Verification items for the finished model (mm, model axes). Give positions to 0.01 mm unless a question says otherwise; leave off trailing zeros. Order: outer loops, then holes, each group sorted by start corner. A loop starts at its lowest first (then second) coordinate and runs counter-clockwise, first axis right, second up. Notation, with made-up numbers: (55, -39) -> (73, -39) arc R18 cw to (73, -12) -> close; hole circle Ø9 at (-3, 67.25). An arc over 180 degrees is marked (long way). Return JSON: item names as keys, results as strings. Group by question number.
(1) Cross-section at B-B on y = 7.5. Enter the section's corners in (x, z) (1 decimal).
(2) Cross-section at A-A on z = 0. Enter the section's corners in (x, y), then the cut area to 3 significant figures.
(3) Thickness scan on line 1 along X through (y, z) = (8.5, -1); line 2 along Z through (x, y) = (-0.25, 5.75); line 3 along X through (y, z) = (9.75, -0.25). Record the ranges inside material, lowest first.
(4) Cross-section at D-D on x = -1.75. Enter the section's corners in (y, z).
(5) Release check for a two-part mould opening along Z. For faces 1 (the face through (1.578, 5.896, -2.784)), 2 (the face through (3.2, 6, 0)), 3 (the face through (-0.31, 5.9, -1.39)) record: pulls with the +Z half, pulls with the -Z half, needs draft (parallel to the pull), parting line crosses it, or undercut.
(6) Depth check by flat-ended pin: pin 1 Ø3 at (x, y) = (-2.5, 6.5) entering from -Z; pin 2 Ø2 at (y, z) = (1.5, -3) entering from +X; pin 3 Ø2 at (x, y) = (2.5, 6.5) entering from -Z. Enter the tip coordinate at first touch or a pass-through.
(7) Cross-section at C-C on x = 0.5. Enter the section's corners in (y, z), then the cut area to 3 significant figures.
Autodesk Inventor part; units mm, degrees
ref_plane "YZ Plane" through (0, 0, 0) normal (1, 0, 0) x (0, 1, 0)
ref_plane "XZ Plane" through (0, 0, 0) normal (0, 1, 0) x (-1, 0, 0)
ref_plane "XY Plane" through (0, 0, 0) normal (0, 0, 1) x (1, 0, 0)
sketch "Sketch1" plane through (0, 0, 0) normal (0, 1, 0) x (-1, 0, 0)
  line L0 (3.2, 1.8475) -> (3.2, -1.8475)
  line L1 (3.2, -1.8475) -> (0, -3.695)
  line L2 (0, -3.695) -> (-3.2, -1.8475)
  line L3 (-3.2, -1.8475) -> (-3.2, 1.8475)
  line L4 (-3.2, 1.8475) -> (0, 3.695)
  line L5 (0, 3.695) -> (3.2, 1.8475)
  point P0 (0, 0)
  point P1 (3.2, 0)
  point P2 (-3.2, 0)
  dimension "d0" = 6.4
  dimension "d1" = 120
  dimension "d2" = 6.4
extrude "Extrusion1" add sketch "Sketch1" along normal blind 11.96
sketch "Sketch3" plane through (0, 0, 0) normal (0, -1, 0) x (1, 0, 0)
  circle A0 centre (0, 0) radius 1.4224
  dimension "d8" = 2.8448
extrude "Extrusion3" cut sketch "Sketch3" against normal through all
properties part number "pc104standoffTEMP2" material "Stainless Steel"
Verdict:
{
 "1": {"outline": "(-3.2, -1.8) -> (0, -3.7) -> (3.2, -1.8) -> (3.2, 1.8) -> (0, 3.7) -> (-3.2, 1.8) -> close; hole circle Ø2.8 at (0, 0)"},
 "2": {"outline": "(-3.2, 0) -> (-1.42, 0) -> (-1.42, 11.96) -> (-3.2, 11.96) -> close; (1.42, 0) -> (3.2, 0) -> (3.2, 11.96) -> (1.42, 11.96) -> close", "area": "42.5 mm²"},
 "3": {"line 1": "-3.2 to -1.01, 1.01 to 3.2", "line 2": "-3.55 to -1.4, 1.4 to 3.55", "line 3": "-3.2 to -1.4, 1.4 to 3.2"},
 "4": {"outline": "(0, -2.68) -> (11.96, -2.68) -> (11.96, 2.68) -> (0, 2.68) -> close"},
 "5": {"face 1": "pulls with the -Z half", "face 2": "needs draft", "face 3": "undercut"},
 "6": {"pin 1": "z = -3.12", "pin 2": "x = 2.94", "pin 3": "z = -2.83"},
 "7": {"outline": "(0, -3.41) -> (11.96, -3.41) -> (11.96, -1.33) -> (0, -1.33) -> close; (0, 1.33) -> (11.96, 1.33) -> (11.96, 3.41) -> (0, 3.41) -> close", "area": "49.6 mm²"}
}
